For this review, take the finished solid that the model builds, in its own axes (mm). A direction names the side the tool comes from. Round coordinates to 2 decimals unless told otherwise and drop trailing zeros. Order: outer loops, then holes, each group sorted by start corner. A loop starts at its lowest first (then second) coordinate and runs counter-clockwise, first axis right, second up. Notation, with made-up numbers: M 80,-37 L 123,-37 A9 ccw 123,-20 Z; hole C 88.25,82.25 d2. An arc over 180 degrees is marked long. Answer as a JSON object with one key per item and string values.
from build123d import *

# Parameters (mm, degrees)
F0_W     = 100
F0_H     = 50
F1_DEPTH = 20
F2_R     = 7
F3_DEPTH = 5
F4_R     = 5
F5_DEPTH = 5
F6_R     = 9
F7_DEPTH = 25


with BuildPart() as f1:
    # F0 (on Top) → F1 (new body)
    with BuildSketch(Plane.XY):
        with Locations((4.46457, -3.417686)):
            Rectangle(F0_W, F0_H)
    extrude(amount=F1_DEPTH)

    # F2 (on face) → F3 (cut)
    with BuildSketch(Plane.XY.offset(20)):
        with Locations((-10.082174, 0)):
            Circle(F2_R)
    extrude(amount=-F3_DEPTH, mode=Mode.SUBTRACT)

    # F4 (on face) → F5 (cut)
    with BuildSketch(Plane.XY.offset(15)):
        with Locations((-10.082174, 0)):
            Circle(F4_R)
    extrude(amount=-F5_DEPTH, mode=Mode.SUBTRACT)

    # F6 (on face) → F7 (cut)
    with BuildSketch(Plane.XY.offset(10)):
        with Locations((-10.082174, 0)):
            Circle(F6_R)
    extrude(amount=-F7_DEPTH, mode=Mode.SUBTRACT)


solid = f1.part
1) Machinability: for faces 1 (the flat face through (-6, -4, 10)), 2 (the flat face through (4, 21.582, 10)), 3 (the flat face through (-15, 2, 15)), which of the approach directions +Z, -Z, +X, -X, +Y, -Y give a long, thin tool a straight path to every point of the face, cutting with its end or side? Answer none if there is none.
Geometry check:
{"face 1": "-Z", "face 2": "+Z, -Z, +X, -X, +Y", "face 3": "+Z"}
2) Add section C-C on z = 12.5. State the section outline as (x, y) points, and give its area (3 significant figures).
Geometry check:
{"outline": "M -45.54,-28.42 L 54.46,-28.42 L 54.46,21.58 L -45.54,21.58 Z; hole C -10.08,0 d10", "area": "4,920 mm²"}
3) For L1, parallel to Y at x = -15, z = 18.5; L2, parallel to Y at x = -13.5, z = 10.25; L3, parallel to X at y = 4, z = 17.5, list the stretches that pass through material, from the lowest coordinate up.
Geometry check:
{"L1": "y = -28.42 to -4.98, 4.98 to 21.58", "L2": "y = -28.42 to -3.65, 3.65 to 21.58", "L3": "x = -45.54 to -15.83, -4.34 to 54.46"}
4) Mouldability with a two-part tool opening along X and no side actions: class faces 4 (the cylindrical face through (-5.313, 1.502, 12.535)), 5 (the flat face through (4, -3, 20)), 6 (the flat face through (54.465, -4, 10)), 7 (the flat face through (-45.535, -4, 10)) as +X half, -X half, draft (parallel to the pull), parting line (faces both ways), or undercut.
Geometry check:
{"face 4": "undercut", "face 5": "draft", "face 6": "+X half", "face 7": "-X half"}
5) Add section A-A on y = 0. State the section outline as (x, z) points.
Geometry check:
{"outline": "M -45.54,0 L -19.08,0 L -19.08,10 L -15.08,10 L -15.08,15 L -17.08,15 L -17.08,20 L -45.54,20 Z; M -5.08,10 L -1.08,10 L -1.08,0 L 54.46,0 L 54.46,20 L -3.08,20 L -3.08,15 L -5.08,15 Z"}
6) Add section B-B on z = 4.75. State the section outline as (x, y) points, and give its area (3 significant figures).
Geometry check:
{"outline": "M -45.54,-28.42 L 54.46,-28.42 L 54.46,21.58 L -45.54,21.58 Z; hole C -10.08,0 d18", "area": "4,750 mm²"}
